Can you work these out from the model? Positions are in its coordinate system, mm. A direction names the side the tool comes from. Coordinates: 2 decimals unless noted, no trailing zeros. Order: outer loops, then holes, each group sorted by start corner. A loop starts at its lowest first (then second) coordinate and runs counter-clockwise, first axis right, second up. Notation, with made-up numbers: (85.25, 5) -> (140.25, 5) arc R28 cw to (140.25, 35) -> close; hole circle Ø8 at (-25.75, -6). An arc over 180 degrees is marked (long way). Answer in a Markdown table with one row per item. Add a question column.
1. Imagine slicing it at A-A on z = 13. Write out the boundary of the cut face in (x, y).
2. Imagine slicing it at D-D on y = 22. Write out the boundary of the cut face in (x, z).
3. Imagine slicing it at B-B on x = 0. Write out the boundary of the cut face in (y, z), plus the area to 3 significant figures.
4. Will these pins go through, and if not, where does the flat tip stop? pin 1 (6.5 mm diameter, centred on y = -2.5, z = -26.5, fed in from -X); pin 2 (10 mm diameter, centred on x = 51.5, y = 2, fed in from -Z); pin 3 (2.5 mm diameter, centred on y = 6, z = 17.5, fed in from +X).
5. If I drill on line 1 along Y through (x, z) = (-55, 16); line 2 along Y through (x, z) = (-10, -19); line 3 along X through (y, z) = (0, 14.25), over which ranges is the centre line in solid material (lowest first)? Write a range as [from, to].
6. We'd pull the mould along Y, two halves only. Please class faces 1 (the face through (-45, 0, 2)), 2 (the face through (47, -30, 10)), 3 (the face through (-32, -1, 15)): pulls with the +Y half, pulls with the -Y half, needs draft (parallel to the pull), parting line crosses it, or undercut.
7. Imagine slicing it at C-C on z = -2. Write out the boundary of the cut face in (x, y), plus the area to 3 significant figures.
8. On a 3-axis mill with a long thin cutter (end or side, diameter ignored), from which of +Z, -Z, +X, -X, +Y, -Y can I reach the whole of each face in a straight line? I mean faces 4 (the face through (-35, -1, 18)), 5 (the face through (-48, -2, 5)), 6 (the face through (-20, 0, -22)), 7 (the face through (-84.993, -0.66, 9.86)), 8 (the face through (66, 0, 0)). Say none if no direction works.
from build123d import *

# Parameters (mm, degrees)
BOSS_EXTRUDE1_DEPTH      = 20
BOSS_EXTRUDE2_DEPTH      = 40
CUT_EXTRUDE1_REACH       = 120.427
SKETCH6_R                = 30
BOSS_EXTRUDE3_REACH      = 108.419
BOSS_EXTRUDE3_END_RADIUS = 40
SKETCH7_W                = 40
SKETCH7_H                = 30
SKETCH7_W_2              = 30
SKETCH7_H_2              = 20
SKETCH8_W                = 70
SKETCH8_H                = 5
CUT_EXTRUDE2_DEPTH       = 121.519707932
HOLE1_D                  = 14
HOLE2_D                  = 14
HOLE2_DEPTH              = 20
HOLE2_CBORE_D            = 20
HOLE2_CBORE_DEPTH        = 5
HOLE2_TIP                = 4.206024333


with BuildPart() as part:
    # Sketch1 → Boss-Extrude1 (new body)
    with BuildSketch(Plane.XY):
        with BuildLine():
            Line((-55, 30), (55, 30))
            ThreePointArc((55, 30), (85, 0), (55, -30))
            Line((55, -30), (-55, -30))
            ThreePointArc((-55, -30), (-85, 0), (-55, 30))
        make_face()
    extrude(amount=BOSS_EXTRUDE1_DEPTH)

    # Sketch5 → Boss-Extrude2 (add, symmetric)
    with BuildSketch(Plane(origin=(0, 0, 0), x_dir=(1, 0, 0), z_dir=(0, 1, 0))):
        with BuildLine():
            Line((-40, -20), (40, -20))
            ThreePointArc((40, -20), (0, 20), (-40, -20))
        make_face()
    extrude(amount=BOSS_EXTRUDE2_DEPTH, both=True)

    # Sketch6 → Cut-Extrude1 (cut, up to next)
    with BuildSketch(Plane(origin=(0, -40, 0), x_dir=(-1, 0, 0), z_dir=(0, -1, 0)), mode=Mode.PRIVATE) as cut_extrude1_sk1:
        with Locations((0, -20)):
            Circle(SKETCH6_R)
    cut_extrude1_tool1 = extrude(cut_extrude1_sk1.sketch, amount=-CUT_EXTRUDE1_REACH, mode=Mode.PRIVATE) & part.part
    add(cut_extrude1_tool1.solids().sort_by_distance((0, -40, 20))[0], mode=Mode.SUBTRACT)

    # Boss-Extrude3: up to this cylinder (the profile starts outside it)
    boss_extrude3_end = Plane(origin=(0, 14.5, 20), z_dir=(0, -1, 0)) * Cylinder(BOSS_EXTRUDE3_END_RADIUS, 297.838, mode=Mode.PRIVATE)
    # Sketch7 → Boss-Extrude3 (add, up to the surface)
    with BuildSketch(Plane(origin=(0, 0, -30), x_dir=(-1, 0, 0), z_dir=(0, 0, -1)), mode=Mode.PRIVATE) as boss_extrude3_sk1:
        Rectangle(SKETCH7_W, SKETCH7_H)
        Rectangle(SKETCH7_W_2, SKETCH7_H_2, mode=Mode.SUBTRACT)
    boss_extrude3_tool1 = extrude(boss_extrude3_sk1.sketch, amount=-BOSS_EXTRUDE3_REACH, mode=Mode.PRIVATE) - boss_extrude3_end
    add(boss_extrude3_tool1.solids().sort_by_distance((0, 14.5, -30))[0])

    # Sketch8 → Cut-Extrude2 (cut, through all)
    with BuildSketch(Plane(origin=(0, -40, 0), x_dir=(-1, 0, 0), z_dir=(0, -1, 0))):
        with Locations((0, -17.5)):
            Rectangle(SKETCH8_W, SKETCH8_H)
    extrude(amount=-CUT_EXTRUDE2_DEPTH, mode=Mode.SUBTRACT)

    # Hole1 (through all)
    with Locations(Plane(origin=(0, 0, -30), x_dir=(-1, 0, 0), z_dir=(0, 0, -1))):
        with Locations((0, 0)):
            Hole(HOLE1_D / 2)

    # Hole2
    with Locations(Plane(origin=(0, 0, 0), x_dir=(-1, 0, 0), z_dir=(0, 0, -1))):
        with Locations((-55, 0), (55, 0)):
            CounterBoreHole(HOLE2_D / 2, HOLE2_CBORE_D / 2, HOLE2_CBORE_DEPTH, depth=HOLE2_DEPTH)
            with Locations((0, 0, -(HOLE2_DEPTH + HOLE2_TIP / 2))):  # 118° drill point
                Cone(0, HOLE2_D / 2, HOLE2_TIP, mode=Mode.SUBTRACT)


solid = part.part
Answers follow:
| question | item | result |
|---|---|---|
| 1 | outline | (-55, -30) -> (-39.38, -30) -> (-39.38, -40) -> (-29.17, -40) -> (-29.17, 40) -> (-39.38, 40) -> (-39.38, 30) -> (-55, 30) arc R30 ccw to start; (29.17, -40) -> (39.38, -40) -> (39.38, -30) -> (55, -30) arc R30 ccw to (55, 30) -> (39.38, 30) -> (39.38, 40) -> (29.17, 40) -> close; hole circle Ø14 at (-55, 0); hole circle Ø14 at (55, 0) |
| 2 | outline | (-75.4, 0) -> (-34.64, 0) arc R40 ccw to (34.64, 0) -> (75.4, 0) -> (75.4, 20) -> (35, 20) -> (35, 15) -> (29.58, 15) arc R30 cw to (-29.58, 15) -> (-35, 15) -> (-35, 20) -> (-75.4, 20) -> close |
| 3 | outline | (-40, -20) -> (-15, -20) -> (-15, -30) -> (-10, -30) -> (-10, -20) -> (-7, -20) -> (-7, -10) -> (-40, -10) -> close; (7, -20) -> (10, -20) -> (10, -30) -> (15, -30) -> (15, -20) -> (40, -20) -> (40, -10) -> (7, -10) -> close |
| 3 | area | 760 mm² |
| 4 | pin 1 | stops at x = -20 |
| 4 | pin 2 | stops at z = 5 |
| 4 | pin 3 | stops at x = 84.62 |
| 5 | line 1 | y = [-30, -7], [7, 30] |
| 5 | line 2 | y = [-15, -10], [10, 15] |
| 5 | line 3 | x = [-85, -62], [-48, -29.44], [29.44, 48], [62, 85] |
| 6 | face 1 | undercut |
| 6 | face 2 | pulls with the -Y half |
| 6 | face 3 | needs draft |
| 7 | outline | (-33.41, -40) -> (-20.4, -40) -> (-20.4, 40) -> (-33.41, 40) -> close; (20.4, -40) -> (33.41, -40) -> (33.41, 40) -> (20.4, 40) -> close |
| 7 | area | 2,080 mm² |
| 8 | face 4 | +Z, +Y, -Y |
| 8 | face 5 | -Z |
| 8 | face 6 | -Z, -X, +Y, -Y |
| 8 | face 7 | +Z, -Z, -X |
| 8 | face 8 | -Z, +X, +Y, -Y |
